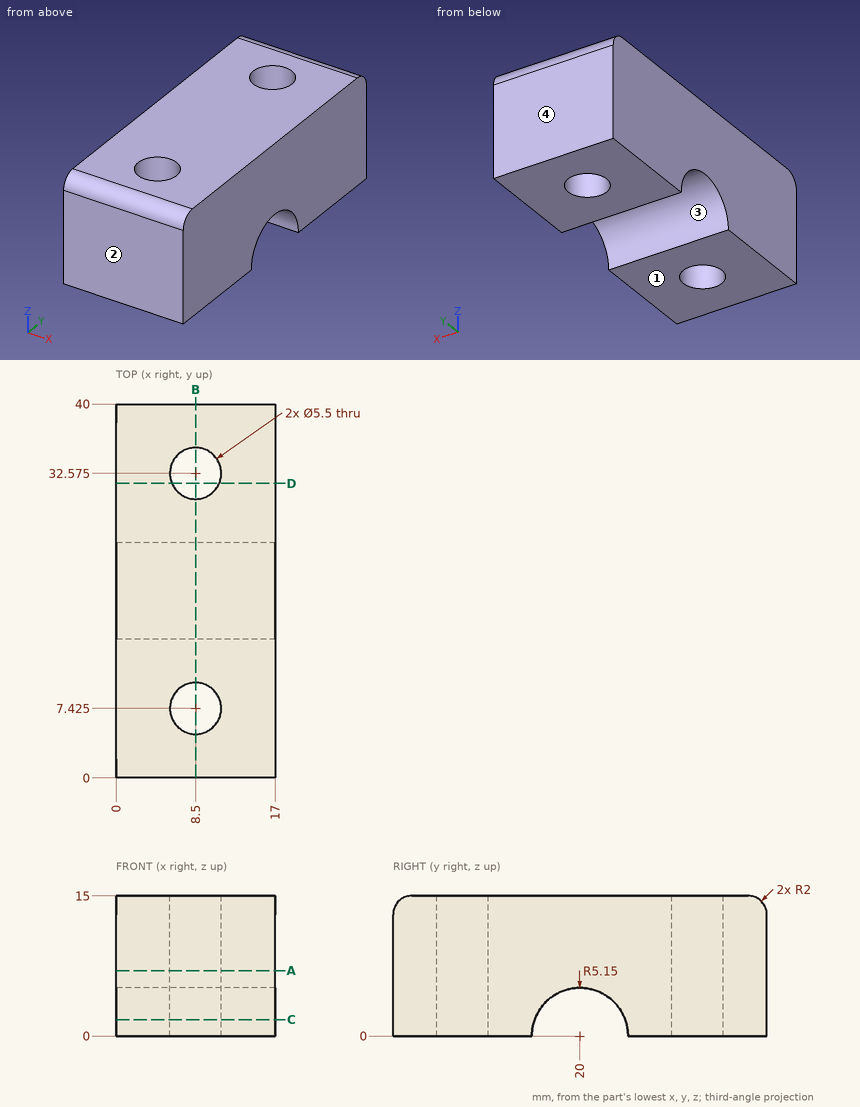
Design review of the part shown in the three views and the two pictorial views. Dimensions are in mm from the part's minimum x, y and z. Coordinates: 2 decimals unless noted, no trailing zeros. Loops run counter-clockwise (first coordinate to the right, second up) from the corner with the lowest first, then second, coordinate; pieces in that order, holes last.
Q1. To check wall thickness, follow line 1 (Y direction, x = 8.5, z = 6.5) (3 decimals); line 2 (Y direction, x = 7.5, z = 1.5); line 3 (Y direction, x = 8.5, z = 3.25) (3 decimals). State the ranges of each line that lie inside material, in increasing order.
Reported:
line 1: y = 0 to 4.675, 10.175 to 29.825, 35.325 to 40
line 2: y = 0 to 4.86, 9.99 to 15.07, 24.93 to 30.01, 35.14 to 40
line 3: y = 0 to 4.675, 10.175 to 16.005, 23.995 to 29.825, 35.325 to 40
Q2. We need section D-D on y = 31.5. State the section outline as (x, z) points.
Reported:
outline: (0, 0) - (5.97, 0) - (5.97, 15) - (0, 15) - close; (11.03, 0) - (17, 0) - (17, 15) - (11.03, 15) - close
Q3. We need section C-C on z = 1.75. State the section outline as (x, y) points (3 decimals).
Reported:
outline: (0, 0) - (17, 0) - (17, 15.156) - (0, 15.156) - close; (0, 24.844) - (17, 24.844) - (17, 40) - (0, 40) - close; hole circle Ø5.5 at (8.5, 7.425); hole circle Ø5.5 at (8.5, 32.575)
Q4. The part is to be moulded in two halves that separate along Y. For the marked faces 1, 2, 3 and 4, say which applies: +Y half, -Y half, draft (parallel to the pull), parting line (faces both ways), or undercut.
Reported:
face 1: draft
face 2: -Y half
face 3: undercut
face 4: +Y half
Q5. We need section A-A on z = 7. State the section outline as (x, y) points (3 decimals).
Reported:
outline: (0, 0) - (17, 0) - (17, 40) - (0, 40) - close; hole circle Ø5.5 at (8.5, 7.425); hole circle Ø5.5 at (8.5, 32.575)
Q6. We need section B-B on x = 8.5. State the section outline as (y, z) points (3 decimals), and give its area (3 significant figures).
Reported:
outline: (0, 0) - (4.675, 0) - (4.675, 15) - (2, 15) arc R2 ccw to (0, 13) - close; (10.175, 0) - (14.85, 0) arc R5.15 cw to (25.15, 0) - (29.825, 0) - (29.825, 15) - (10.175, 15) - close; (35.325, 0) - (40, 0) - (40, 13) arc R2 ccw to (38, 15) - (35.325, 15) - close
area: 392 mm2
